Check sheet for the modelled part. Datum: model origin and axes. Units: mm. A direction names the side the tool comes from. Round coordinates to 2 decimals unless told otherwise and drop trailing zeros. Order: outer loops, then holes, each group sorted by start corner. A loop starts at its lowest first (then second) coordinate and runs counter-clockwise, first axis right, second up. Notation, with made-up numbers: (85.25, 48) -> (103.25, 48) arc R24 cw to (103.25, 59) -> close; hole circle Ø10 at (86.25, 48). An arc over 180 degrees is marked (long way). Answer in a Markdown table with one row per item.
Autodesk Inventor part; units mm, degrees
ref_plane "YZ Plane" through (0, 0, 0) normal (1, 0, 0) x (0, 1, 0)
ref_plane "XZ Plane" through (0, 0, 0) normal (0, 1, 0) x (-1, 0, 0)
ref_plane "XY Plane" through (0, 0, 0) normal (0, 0, 1) x (1, 0, 0)
sketch "Sketch1" plane through (0, 0, 0) normal (0, 1, 0) x (-1, 0, 0)
  point P0 (0, 0)
sketch "Sketch2" plane through (0, 0, 0) normal (0, 1, 0) x (-1, 0, 0)
  line L0 (0, 0) -> (76.2, 0)
  line L1 (76.2, 0) -> (76.2, -115.824)
  line L2 (76.2, -115.824) -> (0, -115.824)
  line L3 (0, -115.824) -> (0, 0)
  dimension "BaseLength" = 76.2
  dimension "BaseWidth" = 115.824
extrude "Base Extrusion" add sketch "Sketch2" along normal blind 6.35
sketch "Sketch3" plane through (0, 0, 0) normal (0, 1, 0) x (-1, 0, 0)
  line L0 (76.2, 0) -> (0, 0)
  line L1 (0, 0) -> (0, -115.824)
  line L2 (0, -115.824) -> (76.2, -115.824)
  line L3 (76.2, -115.824) -> (76.2, 0)
  line L4 (10.8857, 0) -> (21.7714, 0)
  line L5 (21.7714, 0) -> (21.7714, 8.89)
  line L6 (21.7714, 8.89) -> (10.8857, 8.89)
  line L7 (10.8857, 8.89) -> (10.8857, 0)
  line L8 (32.6571, 0) -> (43.5429, 0)
  line L9 (43.5429, 0) -> (43.5429, 8.89)
  line L10 (43.5429, 8.89) -> (32.6571, 8.89)
  line L11 (32.6571, 8.89) -> (32.6571, 0)
  line L12 (54.4286, 0) -> (65.3143, 0)
  line L13 (65.3143, 0) -> (65.3143, 8.89)
  line L14 (65.3143, 8.89) -> (54.4286, 8.89)
  line L15 (54.4286, 8.89) -> (54.4286, 0)
  line L16 (76.2, -57.912) -> (0, -57.912) construction
  line L17 (76.2, -115.824) -> (0, -115.824)
  line L18 (10.8857, -115.824) -> (21.7714, -115.824)
  line L19 (21.7714, -115.824) -> (21.7714, -124.714)
  line L20 (21.7714, -124.714) -> (10.8857, -124.714)
  line L21 (10.8857, -124.714) -> (10.8857, -115.824)
  line L22 (43.5429, -115.824) -> (43.5429, -124.714)
  line L23 (43.5429, -124.714) -> (32.6571, -124.714)
  line L24 (32.6571, -124.714) -> (32.6571, -115.824)
  line L25 (32.6571, -115.824) -> (43.5429, -115.824)
  line L26 (65.3143, -115.824) -> (65.3143, -124.714)
  line L27 (65.3143, -124.714) -> (54.4286, -124.714)
  line L28 (54.4286, -124.714) -> (54.4286, -115.824)
  line L29 (54.4286, -115.824) -> (65.3143, -115.824)
  line L30 (38.1, 0) -> (38.1, -115.824) construction
  line L31 (0, -16.5463) -> (-8.89, -16.5463)
  line L32 (-8.89, -16.5463) -> (-8.89, -33.0926)
  line L33 (-8.89, -33.0926) -> (0, -33.0926)
  line L34 (0, -33.0926) -> (0, -16.5463)
  line L35 (0, -49.6389) -> (-8.89, -49.6389)
  line L36 (-8.89, -49.6389) -> (-8.89, -66.1851)
  line L37 (-8.89, -66.1851) -> (0, -66.1851)
  line L38 (0, -66.1851) -> (0, -49.6389)
  line L39 (0, -82.7314) -> (-8.89, -82.7314)
  line L40 (-8.89, -82.7314) -> (-8.89, -99.2777)
  line L41 (-8.89, -99.2777) -> (0, -99.2777)
  line L42 (0, -99.2777) -> (0, -82.7314)
  line L43 (76.2, 0) -> (76.2, -115.824)
  line L44 (76.2, -16.5463) -> (85.09, -16.5463)
  line L45 (85.09, -16.5463) -> (85.09, -33.0926)
  line L46 (85.09, -33.0926) -> (76.2, -33.0926)
  line L47 (76.2, -33.0926) -> (76.2, -16.5463)
  line L48 (76.2, -49.6389) -> (85.09, -49.6389)
  line L49 (85.09, -49.6389) -> (85.09, -66.1851)
  line L50 (85.09, -66.1851) -> (76.2, -66.1851)
  line L51 (76.2, -66.1851) -> (76.2, -49.6389)
  line L52 (76.2, -82.7314) -> (85.09, -82.7314)
  line L53 (85.09, -82.7314) -> (85.09, -99.2777)
  line L54 (85.09, -99.2777) -> (76.2, -99.2777)
  line L55 (76.2, -99.2777) -> (76.2, -82.7314)
  dimension "d4" = 10.8857
  dimension "d5" = 8.89
  dimension "PerpSpace" = 10.8857
  dimension "d7" = 10.8857
  dimension "d8" = 8.89
  dimension "PerpB" = 10.8857
  dimension "PerpA" = 8.89
  dimension "d11" = 10.8857
  dimension "d13" = 10.8857
  dimension "d14" = 76.2
  dimension "WallConSpace" = 16.5463
  dimension "d16" = 115.824
  dimension "WallConA" = 8.89
  dimension "WallConB" = 16.5463
  dimension "d19" = 8.89
  dimension "d20" = 16.5463
  dimension "d21" = 8.89
  dimension "d22" = 16.5463
  dimension "d23" = 16.5463
  dimension "d24" = 16.5463
extrude "Connections" add sketch "Sketch3" along normal blind 6.35 contours L0 L15 L14 L13 | L44 L45 L46 L3 | L0 L11 L10 L9 | L48 L49 L50 L3 | L0 L7 L6 L5 | L52 L53 L54 L3 | L1 L33 L32 L31 | L26 L27 L28 L2 | L1 L37 L36 L35 | L22 L23 L24 L2 | L1 L41 L40 L39 | L19 L20 L21 L2
equation "\"d4\" = 0.142857 * d14"
equation "\"PerpSpace\" = -0.75 * d4 + 0.25 * d14"
equation "\"d7\" = d4"
equation "\"d8\" = d5"
equation "\"PerpB\" = d4"
equation "\"PerpA\" = d5"
equation "\"d11\" = PerpSpace"
equation "\"d13\" = PerpSpace"
equation "\"WallConSpace\" = -0.75 * WallConB + 0.25 * d16"
equation "\"WallConB\" = 0.142857 * d16"
equation "\"d19\" = WallConA"
equation "\"d20\" = WallConB"
equation "\"d21\" = WallConA"
equation "\"d22\" = WallConB"
equation "\"d23\" = WallConSpace"
equation "\"d24\" = WallConSpace"
properties part number "Level"
(1) Tool access check on faces 4 (the flat face through (-81, 3, -33.093)), 5 (the flat face through (-6, 3, -115.824)), 6 (the flat face through (0, 3, -41)), 7 (the flat face through (-27, 3, 0)). Record the directions out of +Z, -Z, +X, -X, +Y, -Y that give a thin tool (end or side, any length) a straight path to the whole face; none if there is none.
Solutions:
| item | result |
|---|---|
| face 4 | -X, +Y, -Y |
| face 5 | -Z, +X, +Y, -Y |
| face 6 | +X, +Y, -Y |
| face 7 | +Z, +Y, -Y |
(2) Section check B-B on x = -5.5. Record the boundary of the cut face in (y, z), plus the area to 3 significant figures.
Solutions:
| item | result |
|---|---|
| outline | (0, -115.82) -> (6.35, -115.82) -> (6.35, 0) -> (0, 0) -> close |
| area | 735 mm^2 |
(3) Draft check along X on faces 1 (the flat face through (-49, 3, 0)), 2 (the flat face through (-60, 3, -124.714)), 3 (the flat face through (8.89, 3, -25)). Enter one of: pulls with the +X half, pulls with the -X half, needs draft (parallel to the pull), parting line crosses it, or undercut.
Solutions:
| item | result |
|---|---|
| face 1 | undercut |
| face 2 | needs draft |
| face 3 | pulls with the +X half |
(4) Section check A-A on z = -44.5. Record the boundary of the cut face in (x, y), plus the area to 3 significant figures.
Solutions:
| item | result |
|---|---|
| outline | (-76.2, 0) -> (0, 0) -> (0, 6.35) -> (-76.2, 6.35) -> close |
| area | 484 mm^2 |
(5) Depth check by flat-ended pin: pin 1 Ø3 at (y, z) = (2, -122) entering from -X; pin 2 Ø3 at (y, z) = (3.5, 4) entering from +X; pin 3 Ø1.9 at (y, z) = (2.5, -12) entering from +X. Enter the tip coordinate at first touch or a pass-through.
Solutions:
| item | result |
|---|---|
| pin 1 | x = -65.31 |
| pin 2 | x = -10.89 |
| pin 3 | x = 0 |
(6) Scan lines: probe 1 along X at (y, z) = (2, -12.5); probe 2 along Z at (x, y) = (-26.5, 3). Record each from-to range of solid material in increasing order. Write a range as from..to.
Solutions:
| item | result |
|---|---|
| probe 1 | -76.2..0 |
| probe 2 | -115.82..0 |
